The model under review builds one solid part; all positions refer to its coordinate system, in mm. A direction names the side the tool comes from. Round coordinates to 2 decimals unless told otherwise and drop trailing zeros. Order: outer loops, then holes, each group sorted by start corner. A loop starts at its lowest first (then second) coordinate and runs counter-clockwise, first axis right, second up.
```python
from build123d import *

# Parameters (mm, degrees)
SKETCH_1_W          = 100
SKETCH_1_H          = 60
EXTRUDE_1_DEPTH     = 60
SKETCH_2_W          = 94
SKETCH_2_H          = 54
CUT_EXTRUDE_1_DEPTH = 57
CUT_EXTRUDE_2_REACH = 133.149
SKETCH_8_R          = 5.5
SKETCH_9_W          = 106
SKETCH_9_H          = 66
EXTRUDE_2_DEPTH     = 3


with BuildPart() as part:
    # 草图1 → 凸台-拉伸1 (new body)
    with BuildSketch(Plane.XY):
        with Locations((50, 30)):
            Rectangle(SKETCH_1_W, SKETCH_1_H)
    extrude(amount=EXTRUDE_1_DEPTH)

    # 草图2 → 切除-拉伸1 (cut)
    with BuildSketch(Plane.XY.offset(60)):
        with Locations((50, 30)):
            Rectangle(SKETCH_2_W, SKETCH_2_H)
    extrude(amount=-CUT_EXTRUDE_1_DEPTH, mode=Mode.SUBTRACT)

    # 草图8 → 切除-拉伸2 (cut, up to next)
    with BuildSketch(Plane.XZ, mode=Mode.PRIVATE) as cut_extrude_2_sk1:
        with Locations(Location((15, 12, 0), (0, 0, 270))):
            Circle(SKETCH_8_R)
    cut_extrude_2_tool1 = extrude(cut_extrude_2_sk1.sketch, amount=-CUT_EXTRUDE_2_REACH, mode=Mode.PRIVATE) & part.part
    # 草图8 → 切除-拉伸2 (cut, up to next)
    with BuildSketch(Plane.XZ, mode=Mode.PRIVATE) as cut_extrude_2_sk2:
        with Locations(Location((30, 12, 0), (0, 0, 270))):
            Circle(SKETCH_8_R)
    cut_extrude_2_tool2 = extrude(cut_extrude_2_sk2.sketch, amount=-CUT_EXTRUDE_2_REACH, mode=Mode.PRIVATE) & part.part
    add(cut_extrude_2_tool1.solids().sort_by_distance((15, 0, 12))[0], mode=Mode.SUBTRACT)
    add(cut_extrude_2_tool2.solids().sort_by_distance((30, 0, 12))[0], mode=Mode.SUBTRACT)

    # 草图9 → 凸台-拉伸2 (add)
    with BuildSketch(Plane.XY.offset(60)):
        with Locations((50, 30)):
            Rectangle(SKETCH_9_W, SKETCH_9_H)
    extrude(amount=EXTRUDE_2_DEPTH)


solid = part.part
```
(1) Consider section B-B (z = 12). Write out the cut boundary in (x, y), and give its area (3 significant figures).
Data:
outline: (0, 0) - (9.5, 0) - (9.5, 3) - (3, 3) - (3, 57) - (97, 57) - (97, 3) - (35.5, 3) - (35.5, 0) - (100, 0) - (100, 60) - (0, 60) - close; (20.5, 0) - (24.5, 0) - (24.5, 3) - (20.5, 3) - close
area: 858 mm2
(2) Draft analysis for pull direction X (two halves, no side actions). For faces 1 (the flat face through (49, 30, 60)), 2 (the flat face through (49, -3, 61)), 3 (the flat face through (103, 30, 61)), state which applies: pulls with the +X half, pulls with the -X half, needs draft (parallel to the pull), parting line crosses it, or undercut.
Data:
face 1: undercut
face 2: needs draft
face 3: pulls with the +X half
(3) For faces 4 (the cylindrical face through (12.89, 1.48, 6.92)), 5 (the flat face through (49, 60, 30)), 6 (the flat face through (49, 0, 30)), 7 (the flat face through (49, 30, 3)), list the 3-axis set-ups (+Z, -Z, +X, -X, +Y, -Y) from which the entire face can be reached by the end or side of a thin tool; tool diameter is ignored.
Data:
face 4: -Y
face 5: -Z, +X, -X, +Y
face 6: -Z, +X, -X, -Y
face 7: none
(4) Consider section A-A (x = 43). Write out the cut boundary in (y, z), and give its area (3 significant figures).
Data:
outline: (-3, 60) - (0, 60) - (0, 0) - (60, 0) - (60, 60) - (63, 60) - (63, 63) - (-3, 63) - close; hole (3, 3) - (57, 3) - (57, 60) - (3, 60) - close
area: 720 mm2
(5) Consider section D-D (y = 55.5). Write out the cut boundary in (x, z).
Data:
outline: (-3, 60) - (0, 60) - (0, 0) - (100, 0) - (100, 60) - (103, 60) - (103, 63) - (-3, 63) - close; hole (3, 3) - (97, 3) - (97, 60) - (3, 60) - close
(6) To check wall thickness, follow probe 1 along X at (y, z) = (2, 12); probe 2 along Y at (x, z) = (5.5, 15); probe 3 along Z at (x, y) = (88.5, 52.5). State the ranges of each line that lie inside material, in increasing order.
Data:
probe 1: x = 0 to 9.5, 20.5 to 24.5, 35.5 to 100
probe 2: y = 0 to 3, 57 to 60
probe 3: z = 0 to 3, 60 to 63
(7) Insertion check: pin 1 (8 mm diameter, centred on x = 66.5, z = 27.5, fed in from -Y); pin 2 (6.5 mm diameter, centred on x = 30, z = 12, fed in from -Y); pin 3 (1 mm diameter, centred on y = 36.5, z = 42, fed in from +X). Each pin has a flat end and moves straight along its axis. Give the tip position at first contact, or say it passes through.
Data:
pin 1: stops at y = 0
pin 2: stops at y = 57
pin 3: stops at x = 100
(8) Consider section C-C (x = 30). Write out the cut boundary in (y, z).
Data:
outline: (-3, 60) - (0, 60) - (0, 17.5) - (3, 17.5) - (3, 60) - (57, 60) - (57, 3) - (3, 3) - (3, 6.5) - (0, 6.5) - (0, 0) - (60, 0) - (60, 60) - (63, 60) - (63, 63) - (-3, 63) - close
